```python
from build123d import *

# Parameters (mm, degrees)
F1_DEPTH = 25.4
F2_R     = 7.62
F3_R     = 7.62


with BuildPart() as f1:
    # F0 (on Front) → F1 (new body)
    with BuildSketch(Plane.XZ):
        Polygon((-53.984559, -9.564054), (-35.206915, -42.027096), (0.044435, -54.825192), (35.274993, -41.969972), (53.999991, -9.476535), (47.457792, 27.451078), (18.709565, 51.534026), (-18.793075, 51.503631), (-47.502227, 27.374115), align=None)
        Polygon((0.208474, -26.624716), (-16.954337, -20.52972), (-26.184025, -4.82864), (-23.161917, 13.131814), (-9.302091, 24.947747), (8.910288, 25.090351), (22.953443, 13.492902), (26.256428, -4.418027), (17.273738, -20.261711), align=None, mode=Mode.SUBTRACT)
    extrude(amount=F1_DEPTH)

    # F2
    f2_edges = [f1.edges().sort_by_distance(p)[0] for p in [
        (-0.041755, 0, 51.518829),
        (-33.147651, 0, 39.438873),
        (-50.743393, 0, 8.90503),
        (-44.595737, 0, -25.795575),
        (-17.58124, 0, -48.426144),
        (17.659714, 0, -48.397582),
        (44.637492, 0, -25.723254),
        (50.728891, 0, 8.987271),
        (33.083679, 0, 39.492552),
        (-33.147651, -25.4, 39.438873),
        (-0.041755, -25.4, 51.518829),
        (33.083679, -25.4, 39.492552),
        (50.728891, -25.4, 8.987271),
        (44.637492, -25.4, -25.723254),
        (17.659714, -25.4, -48.397582),
        (-17.58124, -25.4, -48.426144),
        (-44.595737, -25.4, -25.795575),
        (-50.743393, -25.4, 8.90503),
    ]]
    fillet(f2_edges, radius=F2_R)

    # F3
    f3_edges = [f1.edges().sort_by_distance(p)[0] for p in [
        (15.931865, -25.4, 19.291626),
        (24.604935, -25.4, 4.537438),
        (21.765083, -25.4, -12.339869),
        (8.741106, -25.4, -23.443213),
        (-8.372932, -25.4, -23.577218),
        (-21.569181, -25.4, -12.67918),
        (-24.672971, -25.4, 4.151587),
        (-16.232004, -25.4, 19.03978),
        (-0.195901, -25.4, 25.019049),
        (-8.372932, 0, -23.577218),
        (8.741106, 0, -23.443213),
        (21.765083, 0, -12.339869),
        (24.604935, 0, 4.537438),
        (15.931865, 0, 19.291626),
        (-0.195901, 0, 25.019049),
        (-16.232004, 0, 19.03978),
        (-24.672971, 0, 4.151587),
        (-21.569181, 0, -12.67918),
    ]]
    fillet(f3_edges, radius=F3_R)


solid = f1.part
```
The model under review builds one solid part; all positions refer to its coordinate system, in mm. A direction names the side the tool comes from. Round coordinates to 2 decimals unless told otherwise and drop trailing zeros. Write each loop counter-clockwise with the first axis right and the second up, starting at its lowest first coordinate (ties: lowest second). Pieces come first, ordered by that corner, then holes.
(1) Machinability: for faces 4 (the flat face through (-32.947, -12.629, 39.608)), 5 (the flat face through (-8.25, -12.63, -23.62)), 6 (the cylindrical face through (26.89, -2.17, 4.79)), which of the approach directions +Z, -Z, +X, -X, +Y, -Y give a long, thin tool a straight path to every point of the face, cutting with its end or side? Answer none if there is none.
(2) Wall thickness on L1, parallel to Z at x = 6.5, y = -12.75; L2, parallel to X at y = -18.25, z = -15.5; L3, parallel to X at y = -22.25, z = 9.5: over which ranges is each line inside the solid? List them lowest first.
(3) Insertion check: pin 1 (3 mm diameter, centred on x = 22, y = -15, fed in from +Z); pin 2 (1 mm diameter, centred on x = -41, z = -19.5, fed in from -Y); pin 3 (1.5 mm diameter, centred on x = -34, z = -35.5, fed in from +Y). Each pin has a flat end and moves straight along its axis. Give the tip position at first contact, or say it passes through.
(4) We need section A-A on y = -13. Give the boundary of the cut face in (x, z) (3 decimals), and give its area (3 significant figures).
(5) We need section B-B on y = -5.75. Give the boundary of the cut face in (x, z), and give its area (3 significant figures).
(6) Mouldability with a two-part tool opening along X and no side actions: class faces 1 (the cylindrical face through (42.9, -2.3, -24.4)), 2 (the cylindrical face through (9.39, -2.17, -25.65)), 3 (the cylindrical face through (-31.951, -23.109, 37.607)) as +X half, -X half, draft (parallel to the pull), parting line (faces both ways), or undercut.
Findings below:
1. face 4: +Z, -X, +Y, -Y
1. face 5: +Y, -Y
1. face 6: +Y
2. L1: z = -52.47 to -24.28, 25.07 to 51.52
2. L2: x = -50.53 to -19.93, 19.99 to 50.51
2. L3: x = -49.17 to -25.24, 25.16 to 49.17
3. pin 1: stops at z = 50.03
3. pin 2: stops at y = -25.35
3. pin 3: stops at y = -0.44
4. outline: (-53.985, -9.564) - (-35.207, -42.027) - (0.044, -54.825) - (35.275, -41.97) - (54, -9.477) - (47.458, 27.451) - (18.71, 51.534) - (-18.793, 51.504) - (-47.502, 27.374) - close; hole (-26.184, -4.829) - (-16.954, -20.53) - (0.208, -26.625) - (17.274, -20.262) - (26.256, -4.418) - (22.953, 13.493) - (8.91, 25.09) - (-9.302, 24.948) - (-23.162, 13.132) - close
4. area: 6,640 mm2
5. outline: (-53.74, -9.52) - (-35.05, -41.84) - (0.04, -54.58) - (35.12, -41.78) - (53.76, -9.43) - (47.24, 27.33) - (18.62, 51.3) - (-18.71, 51.27) - (-47.29, 27.25) - close; hole (-26.43, -4.87) - (-17.11, -20.72) - (0.21, -26.87) - (17.43, -20.45) - (26.5, -4.46) - (23.17, 13.62) - (8.99, 25.32) - (-9.39, 25.18) - (-23.38, 13.25) - close
5. area: 6,530 mm2
6. face 1: +X half
6. face 2: undercut
6. face 3: -X half
